```python
from build123d import *

# Parameters (mm, degrees)
F0_W     = 9.525
F0_H     = 3.175
F0_W_2   = 3.175
F1_DEPTH = 9.525
F2_R     = 1.5875
F3_R     = 1.5875
F4_DEPTH = 25.4


with BuildPart() as f1:
    # F0 (on Top) → F1 (new body)
    with BuildSketch(Plane.XY):
        with Locations((-4.176419, -42.8625)):
            Rectangle(F0_W, F0_H)
        with Locations((2.173581, -42.8625)):
            Rectangle(F0_W_2, F0_H)
        with BuildLine():
            Line((29.161081, -41.275), (32.336081, -41.275))
            ThreePointArc((32.336081, -41.275), (30.476209, -36.784872), (25.986081, -34.925))
            Line((25.986081, -34.925), (6.936081, -34.925))
            ThreePointArc((6.936081, -34.925), (2.445953, -36.784872), (0.586081, -41.275))
            Line((0.586081, -41.275), (3.761081, -41.275))
            ThreePointArc((3.761081, -41.275), (6.936081, -38.1), (10.111081, -41.275))
            ThreePointArc((10.111081, -41.275), (13.286081, -38.1), (16.461081, -41.275))
            ThreePointArc((16.461081, -41.275), (19.636081, -38.1), (22.811081, -41.275))
            ThreePointArc((22.811081, -41.275), (25.986081, -38.1), (29.161081, -41.275))
        make_face()
        with Locations((30.748581, -42.8625)):
            Rectangle(F0_W_2, F0_H)
        with Locations((37.098581, -42.8625)):
            Rectangle(F0_W, F0_H)
    extrude(amount=F1_DEPTH)

    # F2 (on face) + F3 (on face) → F4 (cut)
    with BuildSketch(Plane(origin=(0, -41.275, 0), x_dir=(-1, 0, 0), z_dir=(0, 1, 0))):
        with Locations((4.176419, 4.7625)):
            Circle(F2_R)
    with BuildSketch(Plane(origin=(0, -41.275, 0), x_dir=(-1, 0, 0), z_dir=(0, 1, 0))):
        with Locations((-37.098581, 4.7625)):
            Circle(F3_R)
    extrude(amount=-F4_DEPTH, mode=Mode.SUBTRACT)


solid = f1.part
```
Check sheet for the modelled part. Datum: model origin and axes. Units: mm. A direction names the side the tool comes from. Round coordinates to 2 decimals unless told otherwise and drop trailing zeros. Order: outer loops, then holes, each group sorted by start corner. A loop starts at its lowest first (then second) coordinate and runs counter-clockwise, first axis right, second up.
1) Go/stop test with flat-tipped pins: pin 1 Ø2 at (x, z) = (7, 5.5) entering from -Y; pin 2 Ø3 at (x, z) = (38, 5) entering from +Y (3 decimals). Record where each tip stops, or that it passes through.
2) Section check C-C (z = 5.75). Record the boundary of the cut face in (x, y) (3 decimals), and give its area (3 significant figures).
3) Section check B-B (z = 1.75). Record the boundary of the cut face in (x, y) (3 decimals).
4) Tool access check on faces 4 (the flat face through (-2, -41.275, 5)), 5 (the flat face through (3.761, -43, 5)), 6 (the flat face through (-8.939, -43, 5)), 7 (the flat face through (35, -41.275, 5)). Record the directions out of +Z, -Z, +X, -X, +Y, -Y that give a thin tool (end or side, any length) a straight path to the whole face; none if there is none.
5) Section check D-D (y = -40). Record the boundary of the cut face in (x, z) (3 decimals).
6) Mould release check, pull along X, two halves, no side actions. Record for faces 1 (the cylindrical face through (30.525, -36.835, 4.696)), 2 (the flat face through (29.161, -43, 5)), 3 (the flat face through (35, -44.45, 5)): +X half, -X half, draft (parallel to the pull), parting line (faces both ways), or undercut.
7) Section check A-A (y = -43). Record the boundary of the cut face in (x, z) (1 decimal), and give its area (3 significant figures).
8) Scan lines: line 1 (X direction, y = -44, z = 6.75); line 2 (X direction, y = -38.75, z = 5); line 3 (X direction, y = -39.5, z = 1.25). Record each from-to range of solid material in increasing order.
Result:
1. pin 1: stops at y = -38.28
1. pin 2: stops at y = -41.275
2. outline: (-8.939, -44.45) - (-5.419, -44.45) - (-5.419, -41.275) - (-8.939, -41.275) - close; (-2.933, -44.45) - (3.761, -44.45) - (3.761, -41.275) arc R3.175 cw to (10.111, -41.275) arc R3.175 cw to (16.461, -41.275) arc R3.175 cw to (22.811, -41.275) arc R3.175 cw to (29.161, -41.275) - (29.161, -44.45) - (35.856, -44.45) - (35.856, -41.275) - (32.336, -41.275) arc R6.35 ccw to (25.986, -34.925) - (6.936, -34.925) arc R6.35 ccw to (0.586, -41.275) - (-2.933, -41.275) - close; (38.342, -44.45) - (41.861, -44.45) - (41.861, -41.275) - (38.342, -41.275) - close
2. area: 186 mm2
3. outline: (-8.939, -44.45) - (3.761, -44.45) - (3.761, -41.275) arc R3.175 cw to (10.111, -41.275) arc R3.175 cw to (16.461, -41.275) arc R3.175 cw to (22.811, -41.275) arc R3.175 cw to (29.161, -41.275) - (29.161, -44.45) - (41.861, -44.45) - (41.861, -41.275) - (32.336, -41.275) arc R6.35 ccw to (25.986, -34.925) - (6.936, -34.925) arc R6.35 ccw to (0.586, -41.275) - (-8.939, -41.275) - close
4. face 4: +Z, -Z, -X, +Y
4. face 5: +Z, -Z, -Y
4. face 6: +Z, -Z, -X, +Y, -Y
4. face 7: +Z, -Z, +X, +Y
5. outline: (0.715, 0) - (4.028, 0) - (4.028, 9.525) - (0.715, 9.525) - close; (9.844, 0) - (10.378, 0) - (10.378, 9.525) - (9.844, 9.525) - close; (16.194, 0) - (16.728, 0) - (16.728, 9.525) - (16.194, 9.525) - close; (22.544, 0) - (23.078, 0) - (23.078, 9.525) - (22.544, 9.525) - close; (28.894, 0) - (32.207, 0) - (32.207, 9.525) - (28.894, 9.525) - close
6. face 1: +X half
6. face 2: undercut
6. face 3: draft
7. outline: (-8.9, 0) - (3.8, 0) - (3.8, 9.5) - (-8.9, 9.5) - close; (29.2, 0) - (41.9, 0) - (41.9, 9.5) - (29.2, 9.5) - close; hole circle Ø3.2 at (-4.2, 4.8); hole circle Ø3.2 at (37.1, 4.8)
7. area: 226 mm2
8. line 1: x = -8.94 to 3.76, 29.16 to 41.86
8. line 2: x = 1.11 to 5.01, 8.86 to 11.36, 15.21 to 17.71, 21.56 to 24.06, 27.91 to 31.81
8. line 3: x = 0.84 to 4.3, 9.57 to 10.65, 15.92 to 17, 22.27 to 23.35, 28.62 to 32.08
